Input: dimensioned drawing with shaded views. Units: mm. Origin: part minimum x, y, z. Give positions to 0.01 mm unless a question says otherwise; leave off trailing zeros. Loops run counter-clockwise (first coordinate to the right, second up) from the corner with the lowest first, then second, coordinate; pieces in that order, holes last. Notation, with made-up numbers: M 75.5,50 L 120.5,50 A28 cw 120.5,82 Z; hole C 0.5,62.5 d9. An arc over 180 degrees is marked long. Answer in a Markdown table with one row per item.
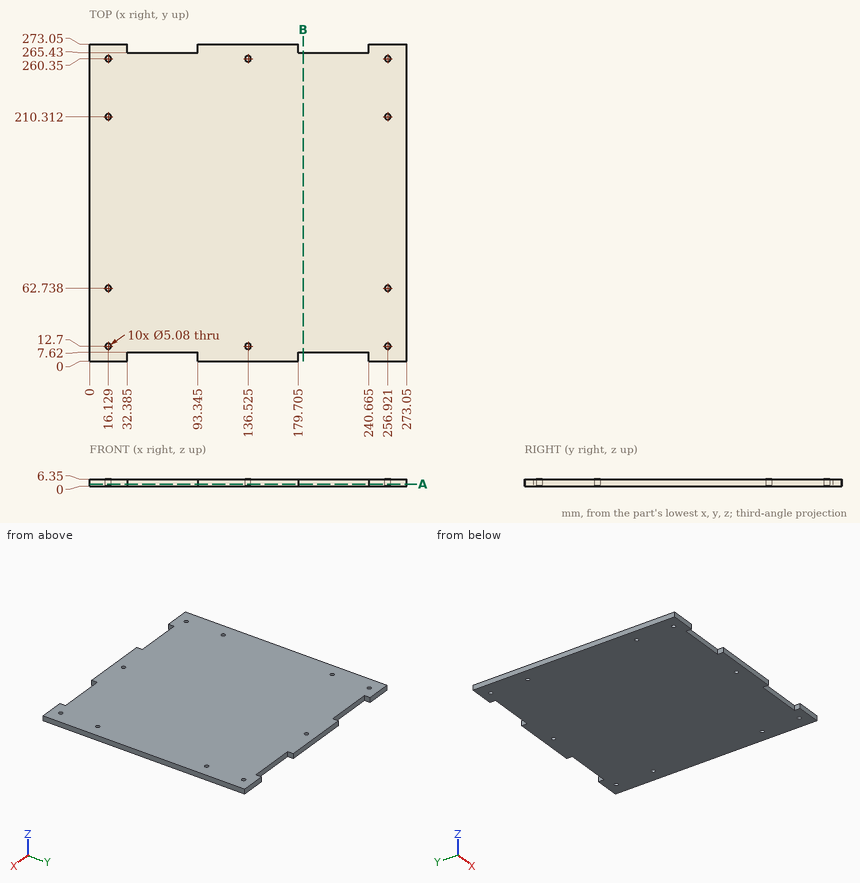
Q1. Section query A-A (z = 2). Give the number of separate pieces and of enclosed holes in the cut face, plus the area to 3 significant figures.
Values follow:
| item | result |
|---|---|
| separate pieces | 1 |
| enclosed holes | 10 |
| area | 72,500 mm^2 |
Q2. Section query B-B (x = 184). Output: boundary loops of the cut face in (y, z), plus the area to 3 significant figures.
Values follow:
| item | result |
|---|---|
| outline | M 7.62,0 L 265.43,0 L 265.43,6.35 L 7.62,6.35 Z |
| area | 1,640 mm^2 |
Q3. Ray query, probe 1 along Y at (x, z) = (136, 5.75); probe 2 along X at (y, z) = (260.35, 3.75) (3 decimals); probe 3 along Y at (x, z) = (257, 1.75). Return the intervals inside material, ascending. Write a range as from..to.
Values follow:
| item | result |
|---|---|
| probe 1 | 0..10.21, 15.19..257.86, 262.84..273.05 |
| probe 2 | 0..13.589, 18.669..133.985, 139.065..254.381, 259.461..273.05 |
| probe 3 | 0..10.16, 15.24..60.2, 65.28..207.77, 212.85..257.81, 262.89..273.05 |
